Read the model definition and answer for the solid it produces. Units are mm, in the model's axes. Coordinates: 2 decimals unless noted, no trailing zeros. Write each loop counter-clockwise with the first axis right and the second up, starting at its lowest first coordinate (ties: lowest second). Pieces come first, ordered by that corner, then holes. Notation, with made-up numbers: (-18.75, 4.25) - (39.25, 4.25) arc R18 cw to (39.25, 12.25) - close; hole circle Ø1 at (88, 15.5). An arc over 180 degrees is marked (long way). Use a Markdown table: item, result.
from build123d import *

# Parameters (mm, degrees)
CROQUIS1_R              = 10
SALIENTE_EXTRUIR1_DEPTH = 148.75
CROQUIS2_W              = 8.300476758
CROQUIS2_H              = 25.089011669
CROQUIS2_W_2            = 8.253581409
CROQUIS2_H_2            = 26.542767485
CORTAR_EXTRUIR1_DEPTH   = 20
CROQUIS3_W              = 10.62874173
CROQUIS3_H              = 2.099903381
CORTAR_EXTRUIR2_DEPTH   = 220
CROQUIS4_R              = 4
CORTAR_EXTRUIR3_DEPTH   = 150.941863734


with BuildPart() as part:
    # Croquis1 → Saliente-Extruir1 (new body)
    with BuildSketch(Plane.XY):
        Circle(CROQUIS1_R)
    extrude(amount=SALIENTE_EXTRUIR1_DEPTH)

    # Croquis2 → Cortar-Extruir1 (cut)
    with BuildSketch(Plane.XY.offset(148.75)):
        with Locations((-10.150238379, -0.750325583)):
            Rectangle(CROQUIS2_W, CROQUIS2_H)
        with Locations((10.126790704, -1.102040699)):
            Rectangle(CROQUIS2_W_2, CROQUIS2_H_2)
    extrude(amount=-CORTAR_EXTRUIR1_DEPTH, mode=Mode.SUBTRACT)

    # Croquis3 → Cortar-Extruir2 (cut)
    with BuildSketch(Plane.XY.offset(148.75)):
        with Locations((-0.162613374, 9.911313118)):
            Rectangle(CROQUIS3_W, CROQUIS3_H)
    extrude(amount=-CORTAR_EXTRUIR2_DEPTH, mode=Mode.SUBTRACT)

    # Croquis4 → Cortar-Extruir3 (cut, through all)
    with BuildSketch(Plane.ZY.offset(6)):
        with Locations(Location((138.75, -0.552617742, 0), (0, 0, 270))):
            Circle(CROQUIS4_R)
    extrude(amount=-CORTAR_EXTRUIR3_DEPTH, mode=Mode.SUBTRACT)


solid = part.part
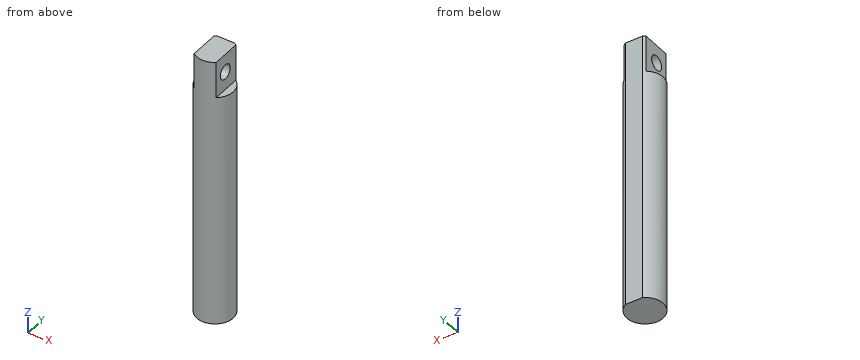
(1) A cutting plane is placed at D-D, the plane y = 6.5. Write down the section's boundary in (x, z), and give its area (3 significant figures).
Report:
| item | result |
|---|---|
| outline | (-7.6, 0) - (7.6, 0) - (7.6, 128.75) - (6, 128.75) - (6, 148.75) - (-6, 148.75) - (-6, 128.75) - (-7.6, 128.75) - close |
| area | 2,200 mm² |
(2) A cutting plane is placed at C-C, the plane y = -1. Write down the section's boundary in (x, z), and give its area (3 significant figures).
Report:
| item | result |
|---|---|
| outline | (-9.95, 0) - (9.95, 0) - (9.95, 128.75) - (6, 128.75) - (6, 134.78) - (-6, 134.78) - (-6, 128.75) - (-9.95, 128.75) - close; (-6, 142.72) - (6, 142.72) - (6, 148.75) - (-6, 148.75) - close |
| area | 2,710 mm² |
(3) A cutting plane is placed at B-B, the plane x = 0. Write down the section's boundary in (y, z).
Report:
| item | result |
|---|---|
| outline | (-10, 0) - (8.86, 0) - (8.86, 148.75) - (-10, 148.75) - close; hole circle Ø8 at (-0.55, 138.75) |
(4) Straight lines are drawn through the part: L1, parallel to Z at x = 6.25, y = 1.75; L2, parallel to Z at x = -4.5, y = -2.25; L3, parallel to Z at x = 3.5, y = -3. For each, find the intervals that lie inside material, in ascending order.
Report:
| item | result |
|---|---|
| L1 | z = 0 to 128.75 |
| L2 | z = 0 to 135.13, 142.37 to 148.75 |
| L3 | z = 0 to 135.59, 141.91 to 148.75 |
(5) A cutting plane is placed at A-A, the plane z = 138.75. Write down the section's boundary in (x, y).
Report:
| item | result |
|---|---|
| outline | (-6, -8) arc R10 ccw to (6, -8) - (6, -4.55) - (-6, -4.55) - close; (-6, 3.45) - (6, 3.45) - (6, 8) arc R10 ccw to (4.63, 8.86) - (-4.63, 8.86) arc R10 ccw to (-6, 8) - close |
(6) Each of these flat-tipped pins is pushed along its axis until it touches: P1, Ø5, axis at y = -2.5, z = 140, coming from the -X side; P2, Ø5, axis at y = -0.55, z = 138.75, coming from the -X side; P3, Ø3, axis at x = -9, y = -3, coming from the +Z side; P4, Ø4, axis at y = -3.5, z = 99, coming from the -X side. Where does it stop, or does it pass through?
Report:
| item | result |
|---|---|
| P1 | stops at x = -6 |
| P2 | passes through |
| P3 | stops at z = 128.75 |
| P4 | stops at x = -9.89 |
